from build123d import *

# Parameters (mm, degrees)
BASE_FLANGE1_DEPTH = 654.05
SKETCH10_W         = 152.4
SKETCH10_H         = 61.9125
CUT_EXTRUDE5_DEPTH = 683.89076222


# Sheet-metal steps are written as plain solids
with BuildPart() as part:
    # Sketch1 → Base-Flange1 (new body)
    with BuildSketch(Plane(origin=(0, 0, 0), x_dir=(0, 0, -1), z_dir=(1, 0, 0))):
        with BuildLine():
            Line((0, 0), (146.05, 0))
            ThreePointArc((146.05, 0), (150.540128061, 1.859871939), (152.4, 6.35))
            Line((152.4, 6.35), (152.4, 117.475))
            ThreePointArc((152.4, 117.475), (150.540128061, 121.965128061), (146.05, 123.825))
            Line((146.05, 123.825), (0, 123.825))
            Line((0, 123.825), (0, 120.65))
            Line((0, 120.65), (146.05, 120.65))
            ThreePointArc((146.05, 120.65), (148.29506403, 119.72006403), (149.225, 117.475))
            Line((149.225, 117.475), (149.225, 6.35))
            ThreePointArc((149.225, 6.35), (148.29506403, 4.10493597), (146.05, 3.175))
            Line((146.05, 3.175), (0, 3.175))
            Line((0, 3.175), (0, 0))
        make_face()
    extrude(amount=BASE_FLANGE1_DEPTH)

    # Sketch10 → Cut-Extrude5 (cut, through all)
    with BuildSketch(Plane(origin=(654.05, 0, 0), x_dir=(0, 0, -1), z_dir=(1, 0, 0))):
        with Locations((76.2, 30.95625)):
            Rectangle(SKETCH10_W, SKETCH10_H)
    extrude(amount=-CUT_EXTRUDE5_DEPTH, mode=Mode.SUBTRACT)


solid = part.part
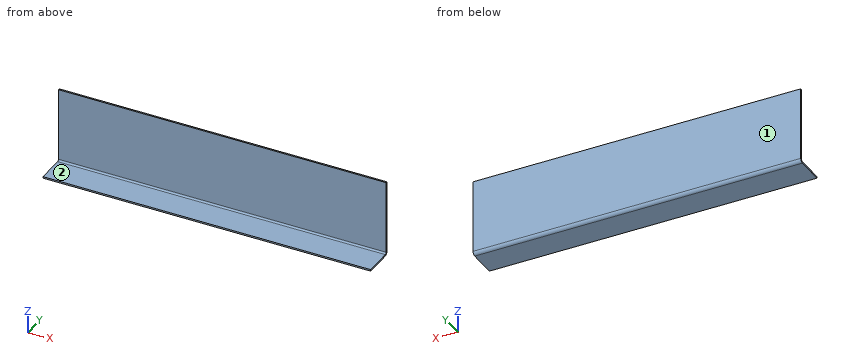
Geometry: final body of the model. Coordinates: model frame, mm. Face numbers are marked on the shaded views. A direction names the side the tool comes from. Give positions to 0.01 mm unless a question says otherwise; leave off trailing zeros. Loops run counter-clockwise (first coordinate to the right, second up) from the corner with the lowest first, then second, coordinate; pieces in that order, holes last. Notation, with made-up numbers: (19.25, -20) -> (60.25, -20) arc R16 cw to (60.25, -3) -> close; hole circle Ø8 at (0.25, -7). An arc over 180 degrees is marked (long way). Put each result on its own line as item: value.
1. Pin query (flat end, axial travel): P1, Ø1, axis at x = 361.5, y = 86, coming from the +Z side (3 decimals). Return the tip coordinate at first contact, or that it passes through.
Taken from the geometry:
P1: stops at z = -149.225
2. Cut plane C-C (y = 93.5). Return the cut outline in (x, z) (3 decimals), plus the area to 3 significant figures.
Taken from the geometry:
outline: (0, -152.4) -> (654.05, -152.4) -> (654.05, -149.225) -> (0, -149.225) -> close
area: 2,080 mm2
3. Set-up query: the marked faces 1 and 2. Return all of +Z, -Z, +X, -X, +Y, -Y with unobstructed straight access to the full face (end or side cutting, diameter ignored); none if empty.
Taken from the geometry:
face 1: +Z, -Z, +X, -X, +Y
face 2: +Z, +X, -X, -Y
4. Ray query, line 1 along Z through (x, y) = (439.5, 116.5) (3 decimals); line 2 along Y through (x, z) = (531.5, -139) (3 decimals); line 3 along Z through (x, y) = (66, 121). Return the intervals inside material, ascending. Write a range as [from, to].
Taken from the geometry:
line 1: z = [-152.4, -149.225]
line 2: y = [120.65, 123.825]
line 3: z = [-151.33, 0]
5. Cut plane B-B (z = -87). Return the cut outline in (x, y) (3 decimals), plus the area to 3 significant figures.
Taken from the geometry:
outline: (0, 120.65) -> (654.05, 120.65) -> (654.05, 123.825) -> (0, 123.825) -> close
area: 2,080 mm2
